Answer from the drawing. Dimensions are ordinates in mm from the lowest x, y and z of the part. A direction names the side the tool comes from. Coordinates: 2 decimals unless noted, no trailing zeros. Loops run counter-clockwise (first coordinate to the right, second up) from the corner with the lowest first, then second, coordinate; pieces in that order, holes last.
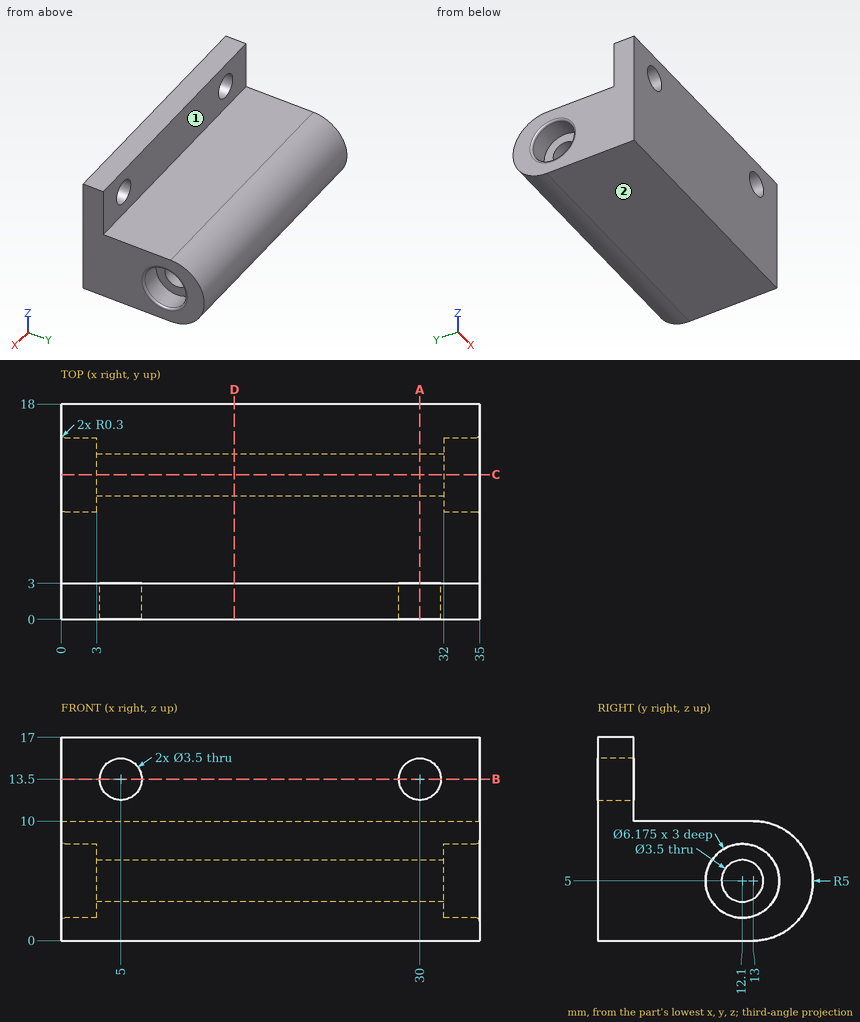
Item 1: Which of the six approach directions +Z, -Z, +X, -X, +Y, -Y give full straight-line access (tool end or side, diameter ignored) to the marked faces 1 and 2?
Numbers:
face 1: +Z, +X, -X, +Y
face 2: -Z, +X, -X, +Y, -Y
Item 2: A cutting plane is placed at D-D on x = 14.5. Determine the outline of the cut face in (y, z), then the cut area to 3 significant figures.
Numbers:
outline: (0, 0) - (13, 0) arc R5 ccw to (13, 10) - (3, 10) - (3, 17) - (0, 17) - close; hole circle Ø3.5 at (12.1, 5)
area: 181 mm2
Item 3: A cutting plane is placed at C-C on y = 12.1. Determine the outline of the cut face in (x, z).
Numbers:
outline: (0, 0) - (35, 0) - (35, 1.61) arc R0.3 ccw to (34.7, 1.91) - (32, 1.91) - (32, 3.25) - (3, 3.25) - (3, 1.91) - (0.3, 1.91) arc R0.3 ccw to (0, 1.61) - close; (0, 8.39) arc R0.3 ccw to (0.3, 8.09) - (3, 8.09) - (3, 6.75) - (32, 6.75) - (32, 8.09) - (34.7, 8.09) arc R0.3 ccw to (35, 8.39) - (35, 10) - (0, 10) - close
Item 4: A cutting plane is placed at A-A on x = 30. Determine the outline of the cut face in (y, z).
Numbers:
outline: (0, 0) - (13, 0) arc R5 ccw to (13, 10) - (3, 10) - (3, 11.75) - (0, 11.75) - close; (0, 15.25) - (3, 15.25) - (3, 17) - (0, 17) - close; hole circle Ø3.5 at (12.1, 5)
Item 5: A cutting plane is placed at B-B on z = 13.5. Determine the outline of the cut face in (x, y).
Numbers:
outline: (0, 0) - (3.25, 0) - (3.25, 3) - (0, 3) - close; (6.75, 0) - (28.25, 0) - (28.25, 3) - (6.75, 3) - close; (31.75, 0) - (35, 0) - (35, 3) - (31.75, 3) - close
Item 6: Given pin 1 (7 mm diameter, centred on y = 12, z = 5, fed in from -X); pin 2 (3 mm diameter, centred on x = 22, z = 9.5, fed in from +Y); pin 3 (3 mm diameter, centred on x = 30, z = 13.5, fed in from +Y); pin 4 (2 mm diameter, centred on x = 15.5, z = 14, fed in from +Y), each flat-ended and moving along its own axis, determine where each tip first touches the part or whether it passes through.
Numbers:
pin 1: stops at x = 0
pin 2: stops at y = 17
pin 3: passes through
pin 4: stops at y = 3
Item 7: Find the intervals of material crossed by line 1 along Y through (x, z) = (1.3, 5); line 2 along X through (y, z) = (1.9, 13.5); line 3 along Z through (x, y) = (2.25, 12.1), in increasing order.
Numbers:
line 1: y = 0 to 9.01, 15.19 to 18
line 2: x = 0 to 3.25, 6.75 to 28.25, 31.75 to 35
line 3: z = 0 to 1.91, 8.09 to 10
